Verification items for this drawing (mm, ordinates from the low corner). A direction names the side the tool comes from. Coordinates: 2 decimals unless noted, no trailing zeros. Order: outer loops, then holes, each group sorted by start corner. A loop starts at its lowest first (then second) coordinate and runs counter-clockwise, first axis right, second up. Notation, with made-up numbers: (89, 11) -> (135, 11) arc R18 ccw to (135, 20) -> close; hole circle Ø5 at (45.5, -33). An arc over 180 degrees is marked (long way). Write item = value, one per line. Start each with the question number.
1. Go/stop test with a flat-tipped pin: P1, Ø1.9, axis at x = 3.5, z = 3, coming from the +Y side. Record where the tip stops, or that it passes through.
2. Cross-section at D-D on x = 0.5. Record the cut outline in (y, z), plus the area to 3 significant figures.
3. Release check for a two-part mould opening along Z. For the marked faces 3, 4 and 5 record: +Z half, -Z half, draft (parallel to the pull), parting line (faces both ways), or undercut.
4. Cross-section at A-A on y = 0.45. Record the cut outline in (x, z) (1 decimal), plus the area to 3 significant figures.
5. Set-up check for the marked faces 1 and 2: record each of +Z, -Z, +X, -X, +Y, -Y from which the full face is reachable in a straight line by a thin tool's end or side.
6. Thickness scan on line 1 along X through (y, z) = (2, 3.2) (1 decimal); line 2 along X through (y, z) = (1.55, 1.5) (1 decimal); line 3 along Z through (x, y) = (2.95, 2.65) (1 decimal). Record the ranges inside material, lowest first. Write a range as from..to.
7. Cross-section at C-C on z = 0.4. Record the cut outline in (x, y).
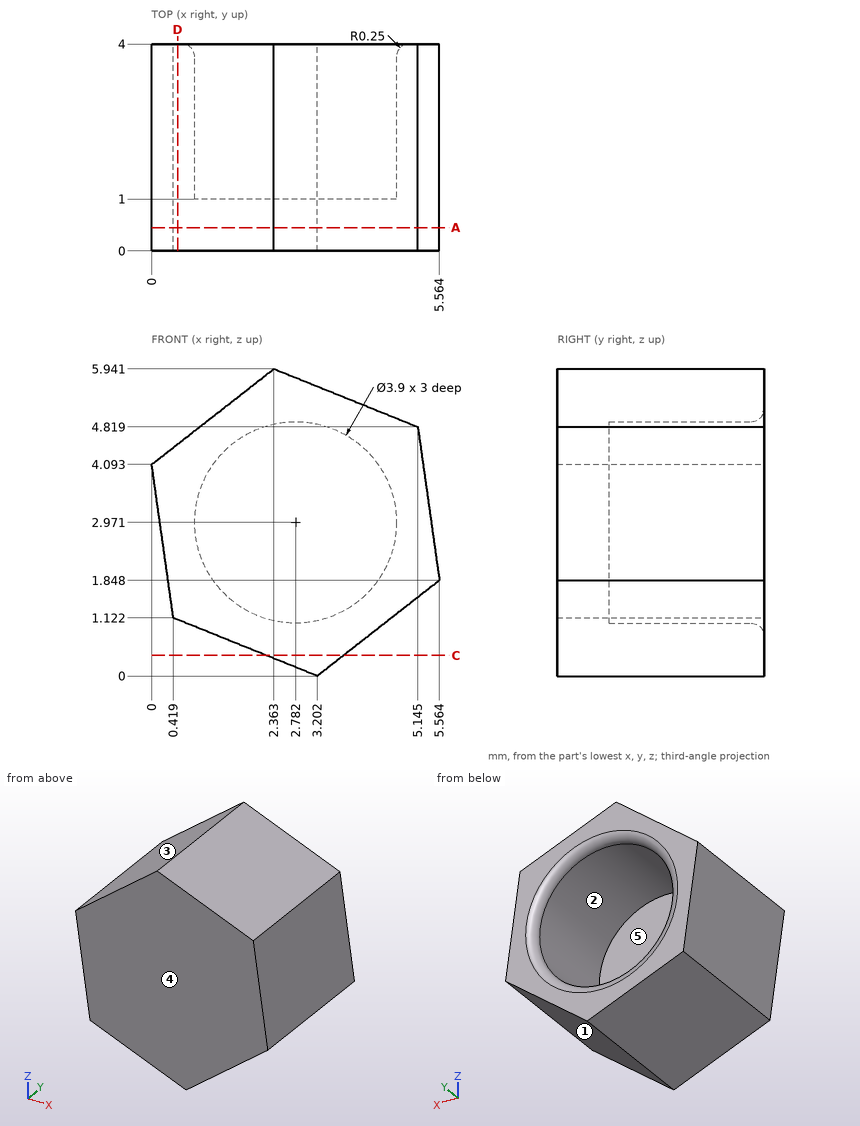
Worked out:
q1.P1 = 1
q2.outline = (0, 1.09) -> (4, 1.09) -> (4, 4.48) -> (0, 4.48) -> close
q2.area = 13.6 mm²
q3.face_3 = +Z half
q3.face_4 = draft
q3.face_5 = undercut
q4.outline = (0, 4.1) -> (0.4, 1.1) -> (3.2, 0) -> (5.6, 1.8) -> (5.1, 4.8) -> (2.4, 5.9) -> close
q4.area = 23.4 mm²
q5.face_1 = -Z, +X, +Y, -Y
q5.face_2 = +Y
q6.line_1 = 0.1..0.8, 4.7..5.4
q6.line_2 = 0.4..1.5, 4.1..5.1
q6.line_3 = 0.1..1, 4.9..5.7
q7.outline = (2.21, 0) -> (3.71, 0) -> (3.71, 4) -> (2.21, 4) -> close
